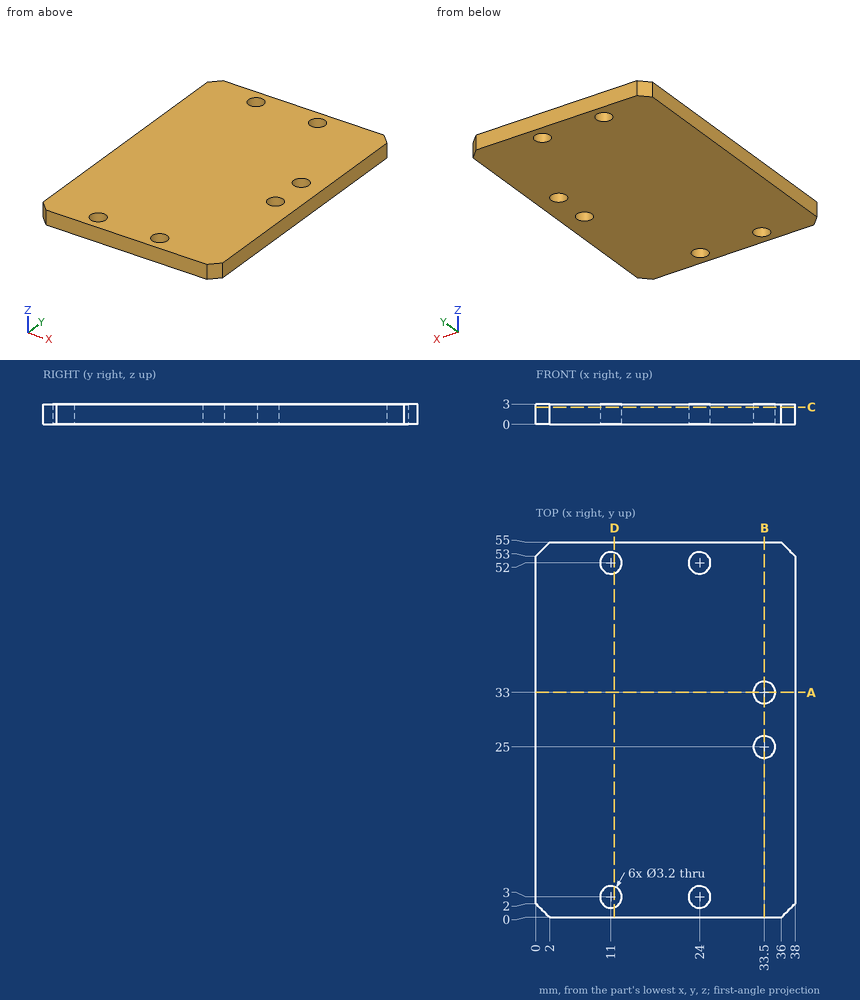
Study the drawing (mm; zero at the part's minimum x, y, z) and answer. Coordinates: 2 decimals unless noted, no trailing zeros. Loops run counter-clockwise (first coordinate to the right, second up) from the corner with the lowest first, then second, coordinate; pieces in that order, holes last. Notation, with made-up numbers: M 45,42.25 L 65,42.25 A14 cw 65,55.25 Z; hole C -31,34.25 d6. An arc over 180 degrees is marked long. Answer as a JSON object with one key per item and string values. Group by question number.
Item 1: Section D-D (x = 11.5) is taken. Write down the section's boundary in (y, z), and give its area (3 significant figures).
Item 2: Each of these flat-tipped pins is pushed along its axis until it touches: P1, Ø1.9, axis at x = 11, y = 52, coming from the -Z side; P2, Ø3.5, axis at x = 33.5, y = 33, coming from the -Z side. Where does it stop, or does it pass through?
Item 3: Section C-C (z = 2.55) is taken. Write down the section's boundary in (x, y).
Item 4: Section B-B (x = 33.5) is taken. Write down the section's boundary in (y, z).
Item 5: Consider L1, parallel to Y at x = 33.5, z = 2.4; L2, parallel to Y at x = 23, z = 2.65. Determine where each line is inside the solid, lowest interval first.
Item 6: Section A-A (y = 33) is taken. Write down the section's boundary in (x, z).
Solved:
{
 "1": {"outline": "M 0,0 L 1.48,0 L 1.48,3 L 0,3 Z; M 4.52,0 L 50.48,0 L 50.48,3 L 4.52,3 Z; M 53.52,0 L 55,0 L 55,3 L 53.52,3 Z", "area": "147 mm2"},
 "2": {"P1": "passes through", "P2": "stops at z = 0"},
 "3": {"outline": "M 0,2 L 2,0 L 36,0 L 38,2 L 38,53 L 36,55 L 2,55 L 0,53 Z; hole C 11,3 d3.2; hole C 11,52 d3.2; hole C 24,3 d3.2; hole C 24,52 d3.2; hole C 33.5,25 d3.2; hole C 33.5,33 d3.2"},
 "4": {"outline": "M 0,0 L 23.4,0 L 23.4,3 L 0,3 Z; M 26.6,0 L 31.4,0 L 31.4,3 L 26.6,3 Z; M 34.6,0 L 55,0 L 55,3 L 34.6,3 Z"},
 "5": {"L1": "y = 0 to 23.4, 26.6 to 31.4, 34.6 to 55", "L2": "y = 0 to 1.75, 4.25 to 50.75, 53.25 to 55"},
 "6": {"outline": "M 0,0 L 31.9,0 L 31.9,3 L 0,3 Z; M 35.1,0 L 38,0 L 38,3 L 35.1,3 Z"}
}
